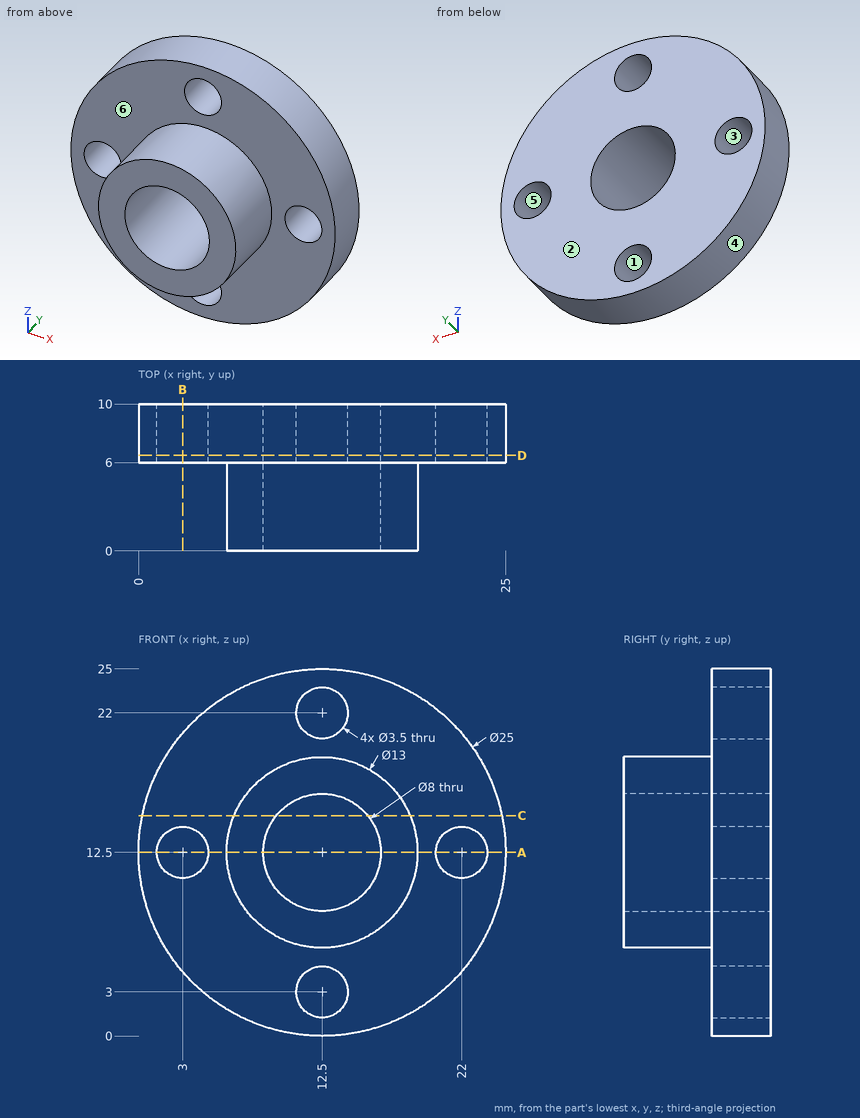
The drawing under review shows one solid part. Ordinate dimensions are in mm from its lowest x, y, z. A direction names the side the tool comes from. Coordinates: 2 decimals unless noted, no trailing zeros. Order: outer loops, then holes, each group sorted by start corner. A loop starts at its lowest first (then second) coordinate and runs counter-clockwise, first axis right, second up. Notation, with made-up numbers: (36, 60) -> (41, 60) arc R17 cw to (41, 91) -> close; hole circle Ø1 at (72, 36). An arc over 180 degrees is marked (long way). Answer in a Markdown table with one row per item. Add a question column.
Item 1: To check wall thickness, follow probe 1 along X at (y, z) = (8.25, 12.5); probe 2 along Z at (x, y) = (12.25, 1.25); probe 3 along X at (y, z) = (4.5, 12.5). State the ranges of each line that lie inside material, in increasing order.
Item 2: We need section A-A on z = 12.5. Write out the cut boundary in (x, y).
Item 3: Mouldability with a two-part tool opening along Z and no side actions: class the marked faces 1, 2, 3 and 4 as +Z half, -Z half, draft (parallel to the pull), parting line (faces both ways), or undercut.
Item 4: We need section D-D on y = 6.5. Write out the cut boundary in (x, z), plus the area to 3 significant figures.
Item 5: Clearance check with flat-ended pins moving along their axes: pin 1 (5.5 mm diameter, centred on x = 12.5, z = 3, fed in from +Y); pin 2 (3 mm diameter, centred on x = 22, z = 12.5, fed in from +Y); pin 3 (2 mm diameter, centred on y = 2.5, z = 7.5, fed in from -X); pin 4 (6 mm diameter, centred on x = 22, y = 5.5, fed in from -Z). State where each tip first meets the part, or that it passes through.
Item 6: We need section B-B on x = 3. Write out the cut boundary in (y, z), plus the area to 3 significant figures.
Item 7: Machinability: for the marked faces 5 and 6, which of the approach directions +Z, -Z, +X, -X, +Y, -Y give a long, thin tool a straight path to every point of the face, cutting with its end or side? Answer none if there is none.
Item 8: We need section C-C on z = 15. Write out the cut boundary in (x, y), plus the area to 3 significant figures.
Final values:
| question | item | result |
|---|---|---|
| 1 | probe 1 | x = 0 to 1.25, 4.75 to 8.5, 16.5 to 20.25, 23.75 to 25 |
| 1 | probe 2 | z = 6 to 8.51, 16.49 to 19 |
| 1 | probe 3 | x = 6 to 8.5, 16.5 to 19 |
| 2 | outline | (0, 6) -> (1.25, 6) -> (1.25, 10) -> (0, 10) -> close; (4.75, 6) -> (6, 6) -> (6, 0) -> (8.5, 0) -> (8.5, 10) -> (4.75, 10) -> close; (16.5, 0) -> (19, 0) -> (19, 6) -> (20.25, 6) -> (20.25, 10) -> (16.5, 10) -> close; (23.75, 6) -> (25, 6) -> (25, 10) -> (23.75, 10) -> close |
| 3 | face 1 | undercut |
| 3 | face 2 | draft |
| 3 | face 3 | undercut |
| 3 | face 4 | parting line |
| 4 | outline | circle Ø25 at (12.5, 12.5); hole circle Ø3.5 at (3, 12.5); hole circle Ø8 at (12.5, 12.5); hole circle Ø3.5 at (12.5, 3); hole circle Ø3.5 at (12.5, 22); hole circle Ø3.5 at (22, 12.5) |
| 4 | area | 402 mm2 |
| 5 | pin 1 | stops at y = 10 |
| 5 | pin 2 | passes through |
| 5 | pin 3 | stops at x = 7.38 |
| 5 | pin 4 | stops at z = 1.85 |
| 6 | outline | (6, 4.38) -> (10, 4.38) -> (10, 10.75) -> (6, 10.75) -> close; (6, 14.25) -> (10, 14.25) -> (10, 20.62) -> (6, 20.62) -> close |
| 6 | area | 51.0 mm2 |
| 7 | face 5 | +Y, -Y |
| 7 | face 6 | -Y |
| 8 | outline | (0.25, 6) -> (6.5, 6) -> (6.5, 0) -> (9.38, 0) -> (9.38, 10) -> (0.25, 10) -> close; (15.62, 0) -> (18.5, 0) -> (18.5, 6) -> (24.75, 6) -> (24.75, 10) -> (15.62, 10) -> close |
| 8 | area | 108 mm2 |
